Autodesk Inventor part; units mm, degrees
ref_plane "Plan YZ" through (0, 0, 0) normal (1, 0, 0) x (0, 1, 0)
ref_plane "Plan XZ" through (0, 0, 0) normal (0, 1, 0) x (-1, 0, 0)
ref_plane "Plan XY" through (0, 0, 0) normal (0, 0, 1) x (1, 0, 0)
sketch "Esquisse1" plane through (0, 0, 0) normal (0, 0, 1) x (1, 0, 0)
  line L0 (-88.5, 55.5) -> (88.5, 55.5)
  line L1 (96.5, 47.5) -> (96.5, -47.5)
  line L2 (88.5, -55.5) -> (-88.5, -55.5)
  line L3 (-96.5, -47.5) -> (-96.5, 47.5)
  line L4 (-170.8, 0) -> (170.8, 0) construction
  line L5 (0, -167.3) -> (0, 104.3) construction
  arc A0 (-88.5, 55.5) -> (-96.5, 47.5) centre (-88.5, 47.5) ccw
  arc A1 (-96.5, -47.5) -> (-88.5, -55.5) centre (-88.5, -47.5) ccw
  arc A2 (88.5, -55.5) -> (96.5, -47.5) centre (88.5, -47.5) ccw
  arc A3 (96.5, 47.5) -> (88.5, 55.5) centre (88.5, 47.5) ccw
  line L6 (-83.4, 49.1) -> (86.6, 49.1) construction
  line L7 (86.6, 49.1) -> (86.6, -51.9) construction
  line L8 (86.6, -51.9) -> (-83.4, -51.9) construction
  line L9 (-83.4, -51.9) -> (-83.4, 49.1) construction
  line L10 (88.5, 52.5) -> (-88.5, 52.5)
  arc A4 (-88.5, 52.5) -> (-93.5, 47.5) centre (-88.5, 47.5) ccw
  line L11 (-93.5, 47.5) -> (-93.5, -47.5)
  arc A5 (-93.5, -47.5) -> (-88.5, -52.5) centre (-88.5, -47.5) ccw
  line L12 (-88.5, -52.5) -> (88.5, -52.5)
  arc A6 (88.5, -52.5) -> (93.5, -47.5) centre (88.5, -47.5) ccw
  line L13 (93.5, -47.5) -> (93.5, 47.5)
  arc A7 (93.5, 47.5) -> (88.5, 52.5) centre (88.5, 47.5) ccw
  line L14 (-122, 65.5) -> (122, 65.5)
  line L15 (122, 65.5) -> (122, -128.5)
  line L16 (122, -128.5) -> (-122, -128.5)
  line L17 (-122, -128.5) -> (-122, 65.5)
  line L18 (122, -31.5) -> (-122, -31.5) construction
  point P0 (0, 0)
  point P1 (-96.5, 55.5)
  point P2 (96.5, -55.5)
  point P3 (96.5, 55.5)
  point P4 (-62.24, 33.92)
  point P5 (-62.24, -31.73)
  point P6 (63.96, -31.73)
  point P7 (63.96, 33.92)
  point P8 (-62.24, 60.5)
  point P9 (-62.24, -60.5)
  point P10 (63.96, -60.5)
  point P11 (63.96, 60.5)
  point P12 (-117, -123.5)
  point P13 (0, -123.5)
  point P14 (117, -123.5)
  point P15 (-117, -31.5)
  point P16 (0, -31.5)
  point P17 (117, -31.5)
  point P18 (-117, 60.5)
  point P19 (0, 60.5)
  point P20 (117, 60.5)
  dimension "d0" = 193
  dimension "d1" = 111
  dimension "d2" = 8
  dimension "d3" = 170
  dimension "d4" = 101
  dimension "d6" = 6.4
  dimension "d7" = 9.9
  dimension "d8" = 32.54
  dimension "d9" = 21.58
  dimension "d10" = 126.2
  dimension "d11" = 65.65
  dimension "d12" = 121
  dimension "d13" = 3
  dimension "d14" = 244
  dimension "d15" = 194
  dimension "d39" = 10
  dimension "d42" = 117
  dimension "d45" = 92
extrude "Extrusion1" add sketch "Esquisse1" along normal blind 3 contours L14 L15 L16 L17
hole "Perçage6" at (-62.24, 33.92, 0) at (-62.24, -31.73, 0) at (63.96, -31.73, 0) at (63.96, 33.92, 0) at (-62.24, 60.5, 0) at (-62.24, -60.5, 0) at (63.96, -60.5, 0) at (63.96, 60.5, 0) at (-117, -123.5, 0) at (0, -123.5, 0) at (117, -123.5, 0) at (-117, -31.5, 0) at (0, -31.5, 0) at (117, -31.5, 0) at (-117, 60.5, 0) at (0, 60.5, 0) at (117, 60.5, 0) direction (0, 0, 1) diameter 3.3 end through all
fillet "Congé1" radius 3 4 edges at (122, -128.5, 1.5) (122, 65.5, 1.5) (-122, 65.5, 1.5) (-122, -128.5, 1.5)
sketch "Esquisse9" plane through (0, 0, 3) normal (0, 0, 1) x (1, 0, 0)
  point P0 (0, 0)
  point P1 (-16, -123)
  point P2 (-16, -64)
  dimension "d66" = 59
  dimension "d67" = 64
  dimension "d68" = 16
hole "Perçage4" at (-16, -123, 3) at (-16, -64, 3) direction (0, 0, -1) diameter 2.2 end through all
properties part number "002" material "Plastique PMMA"
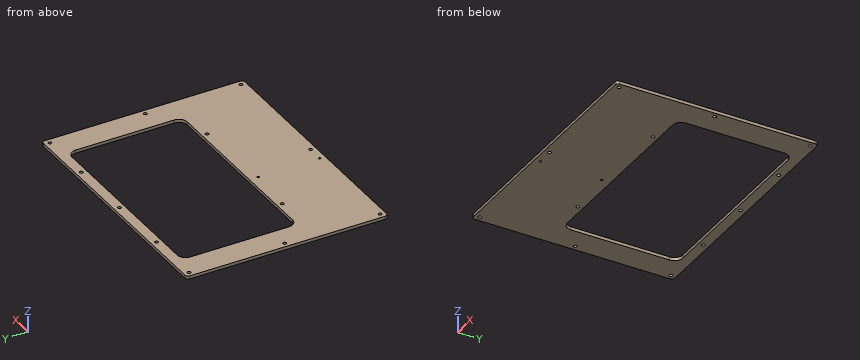
Input: part model. Units: mm. Frame: model coordinates. Coordinates: 2 decimals unless noted, no trailing zeros. Order: outer loops, then holes, each group sorted by start corner. A loop starts at its lowest first (then second) coordinate and runs counter-clockwise, first axis right, second up. Notation, with made-up numbers: M -8.5,-35 L 10.5,-35 A18 ccw 10.5,-27 Z; hole C 35,27 d10. An arc over 180 degrees is marked long. Answer as CSV lines item,"result".
1. First-contact query: P1, Ø2, axis at x = 117, y = -123.5, coming from the -Z side (3 decimals). Flat tip, straight axial feed; report the tip coordinate or a pass-through.
Reported:
P1,"through"
2. Section B-B (y = 3). Return the cut outline in (x, z).
Reported:
outline,"M -122,0 L -96.5,0 L -96.5,3 L -122,3 Z; M 96.5,0 L 122,0 L 122,3 L 96.5,3 Z"
3. Material intervals for line 1 (X direction, y = -60.5, z = 1.5); line 2 (Y direction, x = 117, z = 0.85); line 3 (X direction, y = -31.5, z = 1.65), sorted ascending. Write a range as from..to.
Reported:
line 1,"-122..-63.89, -60.59..62.31, 65.61..122"
line 2,"-128.5..-125.15, -121.85..-33.15, -29.85..58.85, 62.15..65.5"
line 3,"-122..-118.65, -115.35..-96.5, 96.5..115.35, 118.65..122"
4. Section A-A (x = -72.5). Return the cut outline in (y, z).
Reported:
outline,"M -128.5,0 L -55.5,0 L -55.5,3 L -128.5,3 Z; M 55.5,0 L 65.5,0 L 65.5,3 L 55.5,3 Z"
5. Section C-C (z = 0.95). State how many separate pieces and enclosed holes the cut face has, then the cut area to 4 significant figures.
Reported:
separate pieces,"1"
enclosed holes,"15"
area,"25,850 mm2"
